Could you check a few things on this model? Use its own coordinates, in mm. A direction names the side the tool comes from. Round coordinates to 2 decimals unless told otherwise and drop trailing zeros. Order: outer loops, then holes, each group sorted by start corner. A loop starts at its lowest first (then second) coordinate and runs counter-clockwise, first axis right, second up. Notation, with made-up numbers: (76, 78.5) - (124, 78.5) arc R12 cw to (124, 97.5) - close; hole circle Ø9 at (8, 30). An arc over 180 degrees is marked (long way). Return JSON: item names as keys, results as strings. Group by question number.
Autodesk Inventor part; units mm, degrees
ref_plane "YZ Plane" through (0, 0, 0) normal (1, 0, 0) x (0, 1, 0)
ref_plane "XZ Plane" through (0, 0, 0) normal (0, 1, 0) x (-1, 0, 0)
ref_plane "XY Plane" through (0, 0, 0) normal (0, 0, 1) x (1, 0, 0)
sketch "Sketch1" plane through (0, 0, 0) normal (0, 1, 0) x (-1, 0, 0)
  line L0 (-23, 23.29) -> (-23, -23.29)
  line L1 (23, -23.29) -> (23, 23.29)
  line L2 (0, 0) -> (0, -50.5577)
  line L3 (0, 0) -> (-7.5284, 0)
  arc A0 (16.748, -28.1307) -> (-16.748, -28.1307) centre (0, -92.8874) ccw
  arc A1 (-16.748, 28.1307) -> (16.748, 28.1307) centre (0, 92.8874) ccw
  arc A2 (-16.748, 28.1307) -> (-23, 23.29) centre (-18, 23.29) ccw
  arc A3 (-23, -23.29) -> (-16.748, -28.1307) centre (-18, -23.29) ccw
  arc A4 (16.748, -28.1307) -> (23, -23.29) centre (18, -23.29) ccw
  arc A5 (23, 23.29) -> (16.748, 28.1307) centre (18, 23.29) ccw
  line L4 (61.758, -28.29) -> (80.0321, -28.29)
  line L5 (64.4221, 28.29) -> (84.7267, 28.29)
  circle A6 centre (-17.5, -22.5) radius 3.1
  circle A7 centre (17.5, 22.5) radius 3.1
  circle A8 centre (17.5, -22.5) radius 3.1
  circle A9 centre (-17.5, 22.5) radius 3.1
  circle A10 centre (0, 0) radius 8.5
  circle A11 centre (0, 0) radius 4
  dimension "d0" = 52
  dimension "d1" = 46
  dimension "d2" = 5
  dimension "d3" = 56.58
  dimension "d4" = 45
  dimension "d5" = 35
  dimension "d6" = 6.2
  dimension "d9" = 17
  dimension "d15" = 8
extrude "Extrusion1" add sketch "Sketch1" against normal blind 10 contours A2 A1 A5 L1 A4 A0 A3 L0 | L3 A11 L2 | L2 A11 L3 | A6 | A7 | A8 | A9 | A10
extrude "Extrusion2" cut sketch "Sketch1" against normal blind 5 contours L3 A11 L2 | L2 A11 L3 | A10
fillet "Fillet1" radius 4 1 edges at (8.5, 0, 0)
fillet "Fillet2" radius 2 1 edges at (8.5, -5, 0)
shell "Shell1" thickness 1.75 removed faces 9 at (11.424, -10, -7.7633) at (22.3091, -6.6667, 25.8261) at (17.1192, -6.6667, -28.2118) at (-13.0815, -3.3333, 27.2917) at (-13.0815, -6.6667, -27.2917) at (-22.1041, -6.6667, 26.146) at (-22.3091, -6.6667, -25.8261) at (-23, -3.3333, -7.7633) at (23, -3.3333, 7.7633)
extrude "Extrusion3" cut sketch "Sketch1" against normal through all contours L3 A11 L2 | L2 A11 L3 | A6 | A7 | A8 | A9
equation "\"d15\" = 2 * d25"
properties part number "Wheel 75 mm - Part 6"
1) I want a section at A-A, the plane z = 22.5. List the corners of the cut face in (x, y) for me.
2) I want a section at B-B, the plane x = -17.5. List the corners of the cut face in (y, z) for me.
3) For faces 4 (the flat face through (0, -1.75, 13)), 5 (the flat face through (-3, -5, -3)), 6 (the cylindrical face through (-16.828, -0.863, -25.526)), which set-ups out of +Z, -Z, +X, -X, +Y, -Y let a thin tool reach every point of the face, with its end or its side?
4) We'd pull the mould along Z, two halves only. Please class faces 1 (the cylindrical face through (0.867, -5.863, -3.905)), 2 (the flat face through (-3, -6.75, -3)), 3 (the cylindrical face through (21.111, -0.863, -27.204)): +Z half, -Z half, draft (parallel to the pull), parting line (faces both ways), or undercut.
5) If I drill on line 1 along Z through (x, y) = (17.5, -0.95); line 2 along X through (y, z) = (-0.5, 21); line 3 along Z through (x, y) = (-16, -0.75), over which ranges is the centre line in solid material (lowest first)? Write a range as from..to.
6) Will these pins go through, and if not, where does the flat tip stop? pin 1 (1.5 mm diameter, centred on x = 4, y = -1.5, fed in from +Z); pin 2 (3 mm diameter, centred on y = -4.5, z = 7.5, fed in from -X); pin 3 (10.5 mm diameter, centred on x = 0, z = -1, fed in from +Y).
Outcome:
{
 "1": {"outline": "(-23, -1.75) - (-20.6, -1.75) - (-20.6, 0) - (-23, 0) - close; (-14.4, -1.75) - (14.4, -1.75) - (14.4, 0) - (-14.4, 0) - close; (20.6, -1.75) - (23, -1.75) - (23, 0) - (20.6, 0) - close"},
 "2": {"outline": "(-1.75, -28.26) - (0, -28.26) - (0, -25.6) - (-1.75, -25.6) - close; (-1.75, -19.4) - (0, -19.4) - (0, 19.4) - (-1.75, 19.4) - close; (-1.75, 25.6) - (0, 25.6) - (0, 28.26) - (-1.75, 28.26) - close"},
 "3": {"face 4": "-Y", "face 5": "+Y", "face 6": "+Y, -Y"},
 "4": {"face 1": "undercut", "face 2": "draft", "face 3": "-Z half"},
 "5": {"line 1": "-28.26..-25.6, -19.4..19.4, 25.6..28.26", "line 2": "-23..-20.21, -14.79..14.79, 20.21..23", "line 3": "-27.94..-25.21, -19.79..19.79, 25.21..27.94"},
 "6": {"pin 1": "z = 26.17", "pin 2": "x = -8.19", "pin 3": "y = -5"}
}
